from build123d import *

# Parameters (mm, degrees)
F1_DEPTH = 10
F0_R     = 1
F2_START = -8
F0_W     = 2
F0_H     = 0.5
F0_H_2   = 1
F2_DEPTH = 2
F3_DEPTH = 17
F4_R     = 1


with BuildPart() as f1:
    # F0 (on Top) → F1 (new body)
    with BuildSketch(Plane.XY):
        Polygon((35, -2), (35, 2), (28, 2), (28, 0.5), (28, 0), (28, -0.5), (28, -2), align=None)
        with BuildLine():
            ThreePointArc((32.5, 0), (31.5, -1), (30.5, 0))
            ThreePointArc((30.5, 0), (31.5, 1), (32.5, 0))
        make_face(mode=Mode.SUBTRACT)
        with BuildLine():
            ThreePointArc((32.5, 0), (31.5, 1), (30.5, 0))
            ThreePointArc((30.5, 0), (31.5, -1), (32.5, 0))
        make_face()
    extrude(amount=-F1_DEPTH)



with BuildPart() as f1b:
    # F0 (on Top) → F1, piece 2 (new body)
    with BuildSketch(Plane.XY):
        Polygon((-28, 0.5), (-28, 2), (-35, 2), (-35, -2), (-28, -2), (-28, -0.5), align=None)
        with Locations((-31.5, 0)):
            Circle(F0_R, mode=Mode.SUBTRACT)
        with Locations((-31.5, 0)):
            Circle(F0_R)
    extrude(amount=-F1_DEPTH)


with BuildPart() as f1c:
    # F0 (on Top) → F1, piece 3 (new body)
    with BuildSketch(Plane.XY):
        with BuildLine():
            Line((19, -2), (26, -2))
            Line((26, -2), (26, -0.5))
            Line((26, -0.5), (26, 0))
            Line((26, 0), (23.5, 0))
            ThreePointArc((23.5, 0), (22.5, -1), (21.5, 0))
            Line((21.5, 0), (19, 0))
            Line((19, 0), (19, -0.5))
            Line((19, -0.5), (19, -2))
        make_face()
        with BuildLine():
            Line((26, 0.5), (26, 2))
            Line((26, 2), (19, 2))
            Line((19, 2), (19, 0.5))
            Line((19, 0.5), (19, 0))
            Line((19, 0), (21.5, 0))
            ThreePointArc((21.5, 0), (22.5, 1), (23.5, 0))
            Line((23.5, 0), (26, 0))
            Line((26, 0), (26, 0.5))
        make_face()
        with BuildLine():
            Line((22.5, 0), (23.5, 0))
            ThreePointArc((23.5, 0), (22.5, 1), (21.5, 0))
            Line((21.5, 0), (22.5, 0))
        make_face()
        with BuildLine():
            ThreePointArc((21.5, 0), (22.5, -1), (23.5, 0))
            Line((23.5, 0), (22.5, 0))
            Line((22.5, 0), (21.5, 0))
        make_face()
    extrude(amount=-F1_DEPTH)


with BuildPart() as f1d:
    # F0 (on Top) → F1, piece 4 (new body)
    with BuildSketch(Plane.XY):
        with BuildLine():
            Line((10, -2), (17, -2))
            Line((17, -2), (17, -0.5))
            Line((17, -0.5), (17, 0))
            Line((17, 0), (14.5, 0))
            ThreePointArc((14.5, 0), (13.5, -1), (12.5, 0))
            Line((12.5, 0), (10, 0))
            Line((10, 0), (10, -0.5))
            Line((10, -0.5), (10, -2))
        make_face()
        with BuildLine():
            Line((17, 0.5), (17, 2))
            Line((17, 2), (10, 2))
            Line((10, 2), (10, 0.5))
            Line((10, 0.5), (10, 0))
            Line((10, 0), (12.5, 0))
            ThreePointArc((12.5, 0), (13.5, 1), (14.5, 0))
            Line((14.5, 0), (17, 0))
            Line((17, 0), (17, 0.5))
        make_face()
        with BuildLine():
            Line((13.5, 0), (14.5, 0))
            ThreePointArc((14.5, 0), (13.5, 1), (12.5, 0))
            Line((12.5, 0), (13.5, 0))
        make_face()
        with BuildLine():
            ThreePointArc((12.5, 0), (13.5, -1), (14.5, 0))
            Line((14.5, 0), (13.5, 0))
            Line((13.5, 0), (12.5, 0))
        make_face()
    extrude(amount=-F1_DEPTH)


with BuildPart() as f1e:
    # F0 (on Top) → F1, piece 5 (new body)
    with BuildSketch(Plane.XY):
        Polygon((-19, 0.5), (-19, 2), (-26, 2), (-26, 0.5), (-26, -0.5), (-26, -2), (-19, -2), (-19, -0.5), align=None)
        with Locations((-22.5, 0)):
            Circle(F0_R, mode=Mode.SUBTRACT)
        with Locations((-22.5, 0)):
            Circle(F0_R)
    extrude(amount=-F1_DEPTH)


with BuildPart() as f1f:
    # F0 (on Top) → F1, piece 6 (new body)
    with BuildSketch(Plane.XY):
        Polygon((-10, 0.5), (-10, 2), (-17, 2), (-17, 0.5), (-17, -0.5), (-17, -2), (-10, -2), (-10, -0.5), align=None)
        with Locations((-13.5, 0)):
            Circle(F0_R, mode=Mode.SUBTRACT)
        with Locations((-13.5, 0)):
            Circle(F0_R)
    extrude(amount=-F1_DEPTH)


with BuildPart() as f1g:
    # F0 (on Top) → F1, piece 7 (new body)
    with BuildSketch(Plane.XY):
        with BuildLine():
            Line((8, 0.5), (8, 2))
            Line((8, 2), (1, 2))
            Line((1, 2), (1, 0.5))
            Line((1, 0.5), (1, 0))
            Line((1, 0), (3.5, 0))
            ThreePointArc((3.5, 0), (4.5, 1), (5.5, 0))
            Line((5.5, 0), (8, 0))
            Line((8, 0), (8, 0.5))
        make_face()
        with BuildLine():
            Line((1, -2), (8, -2))
            Line((8, -2), (8, -0.5))
            Line((8, -0.5), (8, 0))
            Line((8, 0), (5.5, 0))
            ThreePointArc((5.5, 0), (4.5, -1), (3.5, 0))
            Line((3.5, 0), (1, 0))
            Line((1, 0), (1, -0.5))
            Line((1, -0.5), (1, -2))
        make_face()
        with BuildLine():
            Line((4.5, 0), (5.5, 0))
            ThreePointArc((5.5, 0), (4.5, 1), (3.5, 0))
            Line((3.5, 0), (4.5, 0))
        make_face()
        with BuildLine():
            ThreePointArc((3.5, 0), (4.5, -1), (5.5, 0))
            Line((5.5, 0), (4.5, 0))
            Line((4.5, 0), (3.5, 0))
        make_face()
    extrude(amount=-F1_DEPTH)


with BuildPart() as f1h:
    # F0 (on Top) → F1, piece 8 (new body)
    with BuildSketch(Plane.XY):
        Polygon((-1, 0.5), (-1, 2), (-8, 2), (-8, 0.5), (-8, -0.5), (-8, -2), (-1, -2), (-1, -0.5), align=None)
        with Locations((-4.5, 0)):
            Circle(F0_R, mode=Mode.SUBTRACT)
        with Locations((-4.5, 0)):
            Circle(F0_R)
    extrude(amount=-F1_DEPTH)


with BuildPart() as f1_1:
    add(f1.part)

    add(f1b.part)  # F2 merges F1b

    add(f1c.part)  # F2 merges F1c

    add(f1d.part)  # F2 merges F1d

    add(f1e.part)  # F2 merges F1e

    add(f1f.part)  # F2 merges F1f

    add(f1g.part)  # F2 merges F1g

    add(f1h.part)  # F2 merges F1h
    # F0 (on Top) → F2 (join)
    with BuildSketch(Plane.XY.offset(F2_START)):
        with Locations((9, -0.25)):
            Rectangle(F0_W, F0_H)
        with Locations((9, 0.25)):
            Rectangle(F0_W, F0_H)
        with Locations((18, -0.25)):
            Rectangle(F0_W, F0_H)
        with Locations((18, 0.25)):
            Rectangle(F0_W, F0_H)
        with Locations((27, -0.25)):
            Rectangle(F0_W, F0_H)
        with Locations((27, 0.25)):
            Rectangle(F0_W, F0_H)
        Polygon((1, 0), (1, 0.5), (-1, 0.5), (-1, -0.5), (1, -0.5), align=None)
        with Locations((-9, 0)):
            Rectangle(F0_W, F0_H_2)
        with Locations((-18, 0)):
            Rectangle(F0_W, F0_H_2)
        with Locations((-27, 0)):
            Rectangle(F0_W, F0_H_2)
    extrude(amount=-F2_DEPTH)

    # F0 (on Top) → F3 (join)
    with BuildSketch(Plane.XY):
        with BuildLine():
            ThreePointArc((3.5, 0), (4.5, -1), (5.5, 0))
            Line((5.5, 0), (4.5, 0))
            Line((4.5, 0), (3.5, 0))
        make_face()
        with BuildLine():
            ThreePointArc((12.5, 0), (13.5, -1), (14.5, 0))
            Line((14.5, 0), (13.5, 0))
            Line((13.5, 0), (12.5, 0))
        make_face()
        with BuildLine():
            ThreePointArc((21.5, 0), (22.5, -1), (23.5, 0))
            Line((23.5, 0), (22.5, 0))
            Line((22.5, 0), (21.5, 0))
        make_face()
        with BuildLine():
            ThreePointArc((32.5, 0), (31.5, 1), (30.5, 0))
            ThreePointArc((30.5, 0), (31.5, -1), (32.5, 0))
        make_face()
        with BuildLine():
            Line((22.5, 0), (23.5, 0))
            ThreePointArc((23.5, 0), (22.5, 1), (21.5, 0))
            Line((21.5, 0), (22.5, 0))
        make_face()
        with BuildLine():
            Line((13.5, 0), (14.5, 0))
            ThreePointArc((14.5, 0), (13.5, 1), (12.5, 0))
            Line((12.5, 0), (13.5, 0))
        make_face()
        with BuildLine():
            Line((4.5, 0), (5.5, 0))
            ThreePointArc((5.5, 0), (4.5, 1), (3.5, 0))
            Line((3.5, 0), (4.5, 0))
        make_face()
        with Locations((-4.5, 0)):
            Circle(F0_R)
        with Locations((-13.5, 0)):
            Circle(F0_R)
        with Locations((-22.5, 0)):
            Circle(F0_R)
        with Locations((-31.5, 0)):
            Circle(F0_R)
    extrude(amount=F3_DEPTH)

    # F4
    f4_edges = [f1_1.edges().sort_by_distance(p)[0] for p in [
        (35, 2, -5),
        (28, 2, -5),
        (35, -2, -5),
        (26, 2, -5),
        (19, 2, -5),
        (17, 2, -5),
        (10, 2, -5),
        (8, 2, -5),
        (1, 2, -5),
        (-1, 2, -5),
        (-8, 2, -5),
        (-10, 2, -5),
        (-17, 2, -5),
        (-19, 2, -5),
        (-26, 2, -5),
        (-28, 2, -5),
        (-35, 2, -5),
        (28, -2, -5),
        (26, -2, -5),
        (19, -2, -5),
        (17, -2, -5),
        (10, -2, -5),
        (8, -2, -5),
        (1, -2, -5),
        (-1, -2, -5),
        (-8, -2, -5),
        (-10, -2, -5),
        (-17, -2, -5),
        (-19, -2, -5),
        (-26, -2, -5),
        (-28, -2, -5),
        (-35, -2, -5),
    ]]
    fillet(f4_edges, radius=F4_R)


solid = f1_1.part
Source: CAD feature listing. Evaluate the final solid. Frame: model axes, mm. A direction names the side the tool comes from. Round coordinates to 2 decimals unless told otherwise and drop trailing zeros. Loops run counter-clockwise (first coordinate to the right, second up) from the corner with the lowest first, then second, coordinate; pieces in that order, holes last. Notation, with made-up numbers: (73, -7) - (86, -7) arc R16 cw to (86, 19) - close; hole circle Ø2 at (36, 75). An arc over 180 degrees is marked (long way). Write item = value, one per line. Start each with the question number.
(1) Section query A-A, the plane z = 8.75. Output: boundary loops of the cut face in (x, y).
(2) Section query C-C, the plane z = -6.5. State how many separate pieces and enclosed holes the cut face has, plus the area to 3 significant figures.
(3) Set-up query: faces 3 (the face through (-18, -0.5, -9)), 4 (the face through (-23.5, 0, 8.4)), 5 (the face through (-18, 0.5, -9)). Return all of +Z, -Z, +X, -X, +Y, -Y with unobstructed straight access to the full face (end or side cutting, diameter ignored); none if empty.
(4) Ray query, line 1 along Z through (x, y) = (18, 0.1); line 2 along Z through (x, y) = (-32, -1.45); line 3 along Y through (x, z) = (-5, 12.75). Return the intervals inside material, ascending. Write a range as from..to.
(5) Pin query (flat end, axial travel): pin 1 (12 mm diameter, centred on x = -9.5, z = 14, fed in from -Y); pin 2 (0.5 mm diameter, centred on x = 27, y = 0, fed in from +Z); pin 3 (2 mm diameter, centred on x = 27.5, z = -9, fed in from -Y). Return the tip coordinate at first contact, or that it passes through.
(6) Pull-direction query (X, two-part tool) for faces 1 (the face through (5, 2, -5)), 2 (the face through (1, 0, -5)); classes: +X half, -X half, draft (parallel to the pull), parting line (faces both ways), or undercut.
(7) Section query B-B, the plane x = 4.5. Output: boundary loops of the cut face in (y, z).
Conclusion:
q1.outline = circle Ø2 at (-31.5, 0); circle Ø2 at (-22.5, 0); circle Ø2 at (-13.5, 0); circle Ø2 at (-4.5, 0); circle Ø2 at (4.5, 0); circle Ø2 at (13.5, 0); circle Ø2 at (22.5, 0); circle Ø2 at (31.5, 0)
q2.separate_pieces = 8
q2.enclosed_holes = 0
q2.area = 217 mm2
q3.face_3 = +Z, -Z, -Y
q3.face_4 = +Z
q3.face_5 = +Z, -Z, +Y
q4.line_1 = -10..-8
q4.line_2 = -10..0
q4.line_3 = -0.87..0.87
q5.pin_1 = -1
q5.pin_2 = -8
q5.pin_3 = -1.87
q6.face_1 = draft
q6.face_2 = undercut
q7.outline = (-2, -10) - (2, -10) - (2, 0) - (1, 0) - (1, 17) - (-1, 17) - (-1, 0) - (-2, 0) - close
